Read the model definition and answer for the solid it produces. Units are mm, in the model's axes. Face numbers are marked on the shaded views. Coordinates: 2 decimals unless noted, no trailing zeros. Write each loop counter-clockwise with the first axis right and the second up, starting at its lowest first coordinate (ties: lowest second). Pieces come first, ordered by that corner, then holes. Notation, with made-up numbers: M 29,9 L 67,9 A25 ccw 67,29 Z; hole C 7.25,87 d10. An arc over 180 degrees is marked long. Write item = value, one per line.
from build123d import *
from build123d.topology import SkipClean

# Parameters (mm, degrees)
SKETCH1_R           = 9.652
SKETCH1_R_2         = 19.05
BOSS_EXTRUDE1_DEPTH = 19.05
SKETCH1_3_W         = 57.15
SKETCH1_3_H         = 76.2
BOSS_EXTRUDE2_DEPTH = 57.15
BOSS_EXTRUDE3_DEPTH = 57.15
CUT_EXTRUDE2_DEPTH  = 57.15


with BuildPart() as part:
    # Sketch1 → Boss-Extrude1 (new body)
    with BuildSketch(Plane(origin=(0, 0, 0), x_dir=(1, 0, 0), z_dir=(0, 1, 0))):
        with BuildLine():
            ThreePointArc((-349.25, -101.6), (-341.810512242, -119.560512242), (-323.85, -127))
            Line((-323.85, -127), (323.85, -127))
            ThreePointArc((323.85, -127), (341.810512242, -119.560512242), (349.25, -101.6))
            Line((349.25, -101.6), (349.25, -38.1))
            Line((349.25, -38.1), (292.1, -38.1))
            Line((292.1, -38.1), (292.1, 38.1))
            Line((292.1, 38.1), (349.25, 38.1))
            Line((349.25, 38.1), (349.25, 101.6))
            ThreePointArc((349.25, 101.6), (341.810512242, 119.560512242), (323.85, 127))
            Line((323.85, 127), (-323.85, 127))
            ThreePointArc((-323.85, 127), (-341.810512242, 119.560512242), (-349.25, 101.6))
            Line((-349.25, 101.6), (-349.25, 38.1))
            Line((-349.25, 38.1), (-292.1, 38.1))
            Line((-292.1, 38.1), (-292.1, -38.1))
            Line((-292.1, -38.1), (-349.25, -38.1))
            Line((-349.25, -38.1), (-349.25, -101.6))
        make_face()
        with Locations(Location((-323.85, -101.6, 0), (0, 0, 90))):
            Circle(SKETCH1_R, mode=Mode.SUBTRACT)
        with Locations(Location((323.85, -101.6, 0), (0, 0, 90))):
            Circle(SKETCH1_R, mode=Mode.SUBTRACT)
        with Locations(Location((-323.85, 101.6, 0), (0, 0, 90))):
            Circle(SKETCH1_R, mode=Mode.SUBTRACT)
        with Locations(Location((0, 0, 0), (0, 0, 90))):
            Circle(SKETCH1_R_2, mode=Mode.SUBTRACT)
        with Locations(Location((323.85, 101.6, 0), (0, 0, 90))):
            Circle(SKETCH1_R, mode=Mode.SUBTRACT)
    extrude(amount=BOSS_EXTRUDE1_DEPTH)

    # Sketch1_3 → Boss-Extrude2 (add)
    with BuildSketch(Plane(origin=(0, 0, 0), x_dir=(1, 0, 0), z_dir=(0, 1, 0))):
        with Locations((-320.675, 0)):
            Rectangle(SKETCH1_3_W, SKETCH1_3_H)
        with Locations((320.675, 0)):
            Rectangle(SKETCH1_3_W, SKETCH1_3_H)
    extrude(amount=BOSS_EXTRUDE2_DEPTH)

    # Sketch2 → Boss-Extrude3 (add)
    with BuildSketch(Plane(origin=(349.25, 0, 0), x_dir=(0, 0, -1), z_dir=(1, 0, 0))):
        with BuildLine():
            Line((19.05, 57.15), (38.1, 57.15))
            ThreePointArc((38.1, 57.15), (0, 95.25), (-38.1, 57.15))
            Line((-38.1, 57.15), (-19.05, 57.15))
            ThreePointArc((-19.05, 57.15), (0, 76.2), (19.05, 57.15))
        make_face()
    boss_extrude3 = extrude(amount=-BOSS_EXTRUDE3_DEPTH)

    # Sketch2_4 → Cut-Extrude2 (cut)
    with BuildSketch(Plane(origin=(349.25, 0, 0), x_dir=(0, 0, -1), z_dir=(1, 0, 0))):
        with BuildLine():
            ThreePointArc((-19.05, 57.15), (0, 38.1), (19.05, 57.15))
            Line((19.05, 57.15), (-19.05, 57.15))
        make_face()
        with BuildLine():
            Line((-19.05, 57.15), (19.05, 57.15))
            ThreePointArc((19.05, 57.15), (0, 76.2), (-19.05, 57.15))
        make_face()
    cut_extrude2 = extrude(amount=-CUT_EXTRUDE2_DEPTH, mode=Mode.SUBTRACT)

    # Mirror1: Boss-Extrude3, Cut-Extrude2 across plane
    with SkipClean():  # the faces are left unmerged after this step: merging them gives an invalid solid
        add(boss_extrude3.mirror(Plane(origin=(0, 0, 0), x_dir=(0, 0, 1), z_dir=(1, 0, 0))))
        add(cut_extrude2.mirror(Plane(origin=(0, 0, 0), x_dir=(0, 0, 1), z_dir=(1, 0, 0))), mode=Mode.SUBTRACT)


solid = part.part
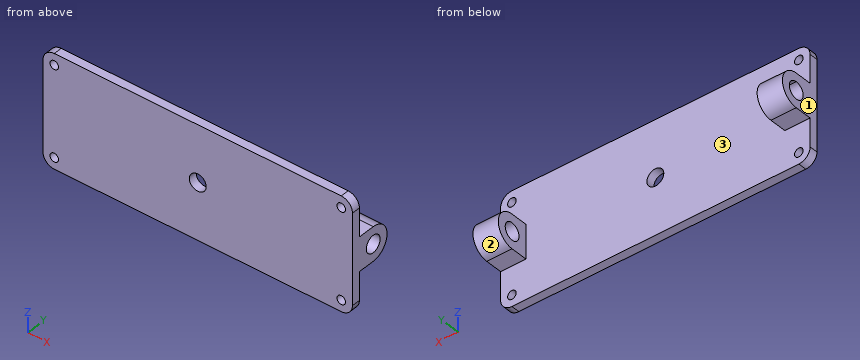
Item 1: Find section B-B (y = 29). Determine the outline of the cut face in (x, z), and give its area (3 significant figures).
Worked answers:
outline = M -349.25,-38.1 L -292.1,-38.1 L -292.1,38.1 L -349.25,38.1 Z; M 292.1,-38.1 L 349.25,-38.1 L 349.25,38.1 L 292.1,38.1 Z
area = 8,710 mm²
Item 2: Find section D-D (x = 198.5). Determine the outline of the cut face in (y, z), and give its area (3 significant figures).
Worked answers:
outline = M 0,-127 L 19.05,-127 L 19.05,127 L 0,127 Z
area = 4,840 mm²
Item 3: Consider line 1 along Z through (x, y) = (-323, 14); line 2 along Z through (x, y) = (-323.85, 7.5); line 3 along X through (y, z) = (4, -101). Determine where each line is inside the solid, lowest interval first. Write a range as from..to.
Worked answers:
line_1 = -127..-111.21, -91.99..91.99, 111.21..127
line_2 = -127..-111.25, -91.95..91.95, 111.25..127
line_3 = -349.25..-333.48, -314.22..314.22, 333.48..349.25
Item 4: Find section C-C (z = 0). Determine the outline of the cut face in (x, y), and give its area (3 significant figures).
Worked answers:
outline = M -349.25,0 L -19.05,0 L -19.05,19.05 L -292.1,19.05 L -292.1,38.1 L -349.25,38.1 Z; M -349.25,76.2 L -292.1,76.2 L -292.1,95.25 L -349.25,95.25 Z; M 19.05,0 L 349.25,0 L 349.25,38.1 L 292.1,38.1 L 292.1,19.05 L 19.05,19.05 Z; M 292.1,76.2 L 349.25,76.2 L 349.25,95.25 L 292.1,95.25 Z
area = 16,900 mm²
Item 5: Flat-ended cylindrical pins translate along their axes: pin 1 (11.5 mm diameter, centred on x = -323.85, z = -101.6, fed in from -Y); pin 2 (11.5 mm diameter, centred on x = -317, y = 39, fed in from -Z); pin 3 (11.5 mm diameter, centred on x = 325.5, y = 45, fed in from +Z). Find the tip coordinate at first contact, or state that the pin passes through.
Worked answers:
pin_1 = through
pin_2 = -38.1
pin_3 = 38.1
Item 6: Find section A-A (x = 0). Determine the outline of the cut face in (y, z), and give its area (3 significant figures).
Worked answers:
outline = M 0,-127 L 19.05,-127 L 19.05,-19.05 L 0,-19.05 Z; M 0,19.05 L 19.05,19.05 L 19.05,127 L 0,127 Z
area = 4,110 mm²
Item 7: For a pull along X with two mould halves and no side action, classify the marked faces 1, 2 and 3 as released by +X, released by -X, zero draft, split by the parting line, or undercut.
Worked answers:
face_1 = released by -X
face_2 = zero draft
face_3 = undercut
